Source: CAD feature listing. Evaluate the final solid. Frame: model axes, mm. Coordinates: 2 decimals unless noted, no trailing zeros. Write each loop counter-clockwise with the first axis right and the second up, starting at its lowest first coordinate (ties: lowest second). Pieces come first, ordered by that corner, then holes. Notation, with made-up numbers: (-21.5, 85.5) -> (24.5, 85.5) arc R14 ccw to (24.5, 103.5) -> close; hole circle Ø6 at (46, 66.25). An arc over 180 degrees is marked (long way). Write item = value, one per line.
from build123d import *

# Parameters (mm, degrees)
SKETCH1_R           = 12.0000014
SKETCH1_R_2         = 29.99994
SKETCH1_R_3         = 15.99946
BOSS_EXTRUDE1_DEPTH = 19.05


with BuildPart() as part:
    # Sketch1 → Boss-Extrude1 (new body)
    with BuildSketch(Plane.XY):
        with BuildLine():
            Line((1666.449914345, 1807.663309633), (1666.449914345, 984.292129537))
            add(Edge.make_bspline(
                [(1860.24643809, 984.292129537), (1834.442562073, 925.070762843), (1666.449914345, 919.693288289), (1666.449914345, 984.292129537)],
                knots=[0, 0, 0, 0, 7.629784399, 7.629784399, 7.629784399, 7.629784399], degree=3))
            ThreePointArc((1860.24643809, 984.292129537), (1946.092561687, 1395.955210336), (1860.46260196, 1807.663309633))
            add(Edge.make_bspline(
                [(1860.46260196, 1807.663309633), (1834.661077492, 1866.964288613), (1666.449914345, 1872.334205504), (1666.449914345, 1807.663309633)],
                knots=[0, 0, 0, 0, 7.638294788, 7.638294788, 7.638294788, 7.638294788], degree=3))
        make_face()
        with Locations(Location((1811.402116463, 1181.948319082, 0), (0, 0, 180))):
            Circle(SKETCH1_R, mode=Mode.SUBTRACT)
        with Locations(Location((1820.402123863, 1146.948389082, 0), (0, 0, 180))):
            Circle(SKETCH1_R, mode=Mode.SUBTRACT)
        with Locations(Location((1838.402113263, 1115.698388082, 0), (0, 0, 180))):
            Circle(SKETCH1_R, mode=Mode.SUBTRACT)
        with Locations(Location((1772.402194463, 1146.948389082, 0), (0, 0, 180))):
            Circle(SKETCH1_R, mode=Mode.SUBTRACT)
        with Locations(Location((1790.402183863, 1115.698388082, 0), (0, 0, 180))):
            Circle(SKETCH1_R, mode=Mode.SUBTRACT)
        with Locations(Location((1763.402187063, 1181.948319082, 0), (0, 0, 180))):
            Circle(SKETCH1_R, mode=Mode.SUBTRACT)
        with Locations(Location((1818.401594463, 1051.948325082, 0), (0, 0, 180))):
            Circle(SKETCH1_R, mode=Mode.SUBTRACT)
        with Locations(Location((1811.402116463, 1723.918527241, 0), (0, 0, 180))):
            Circle(SKETCH1_R, mode=Mode.SUBTRACT)
        with Locations(Location((1820.402123863, 1688.918597241, 0), (0, 0, 180))):
            Circle(SKETCH1_R, mode=Mode.SUBTRACT)
        with Locations(Location((1838.402113263, 1657.668596241, 0), (0, 0, 180))):
            Circle(SKETCH1_R, mode=Mode.SUBTRACT)
        with Locations(Location((1772.402194463, 1688.918597241, 0), (0, 0, 180))):
            Circle(SKETCH1_R, mode=Mode.SUBTRACT)
        with Locations(Location((1790.402183863, 1657.668596241, 0), (0, 0, 180))):
            Circle(SKETCH1_R, mode=Mode.SUBTRACT)
        with Locations(Location((1763.402187063, 1723.918527241, 0), (0, 0, 180))):
            Circle(SKETCH1_R, mode=Mode.SUBTRACT)
        with Locations(Location((1818.401594463, 1593.918533241, 0), (0, 0, 180))):
            Circle(SKETCH1_R, mode=Mode.SUBTRACT)
        with Locations(Location((1788.861738175, 1363.125382024, 0), (0, 0, 180))):
            Circle(SKETCH1_R, mode=Mode.SUBTRACT)
        with Locations(Location((1789.336065957, 1426.620354396, 0), (0, 0, 180))):
            Circle(SKETCH1_R, mode=Mode.SUBTRACT)
        with Locations(Location((1857.192561687, 1395.955210336, 0), (0, 0, 180))):
            Circle(SKETCH1_R_2, mode=Mode.SUBTRACT)
        with Locations(Location((1714.690199276, 1395.955210336, 0), (0, 0, 180))):
            Circle(SKETCH1_R_3, mode=Mode.SUBTRACT)
    extrude(amount=BOSS_EXTRUDE1_DEPTH)


solid = part.part
1) Pull-direction query (X, two-part tool) for faces 1 (the flat face through (1666.45, 1402, 9)), 2 (the cylindrical face through (1798.38, 1370.43, 9.39)), 3 (the cylindrical face through (1946.074, 1390.026, 9.392)), 4 (the flat face through (1773, 1403, 0)); classes: +X half, -X half, draft (parallel to the pull), parting line (faces both ways), or undercut.
Answer block:
face_1 = -X half
face_2 = undercut
face_3 = +X half
face_4 = draft
2) Cut plane A-A, the plane z = 5.25. Give the number of separate pieces and of enclosed holes in the cut face, and give its area (3 significant figures).
Answer block:
separate_pieces = 1
enclosed_holes = 18
area = 210,000 mm2
3) Material intervals for probe 1 along X at (y, z) = (1678.5, 12.5); probe 2 along Y at (x, z) = (1797, 17); probe 3 along Y at (x, z) = (1792, 1.75), sorted ascending. Write a range as [from, to].
Answer block:
probe_1 = [1666.45, 1766.45], [1778.36, 1814.45], [1826.36, 1906.71]
probe_2 = [943.24, 1105.67], [1125.72, 1354.31], [1371.94, 1417.39], [1435.85, 1647.65], [1667.69, 1848.81]
probe_3 = [942.11, 1103.81], [1127.59, 1351.54], [1374.71, 1414.92], [1438.32, 1645.78], [1669.56, 1849.93]
4) First-contact query: pin 1 Ø14.5 at (x, y) = (1772.4, 1688.92) entering from -Z; pin 2 Ø10 at (x, z) = (1726.5, 17) entering from +Y; pin 3 Ø10 at (x, z) = (1820.5, 9) entering from +Y; pin 4 Ø3 at (x, z) = (1711.5, 14) entering from -Y. Flat tips, straight axial feed; report the tip coordinate or a pass-through.
Answer block:
pin_1 = through
pin_2 = 1853.18
pin_3 = 1843.23
pin_4 = 941.92
5) Cut plane B-B, the plane y = 1295.5. Output: boundary loops of the cut face in (x, z), and give its area (3 significant figures).
Answer block:
outline = (1666.45, 0) -> (1941.16, 0) -> (1941.16, 19.05) -> (1666.45, 19.05) -> close
area = 5,230 mm2
6) Cut plane C-C, the plane x = 1924.5. Output: boundary loops of the cut face in (y, z), and give its area (3 significant figures).
Answer block:
outline = (1186.3, 0) -> (1606.15, 0) -> (1606.15, 19.05) -> (1186.3, 19.05) -> close
area = 8,000 mm2
